Read the model definition and answer for the solid it produces. Units are mm, in the model's axes. A direction names the side the tool comes from. Coordinates: 2 decimals unless noted, no trailing zeros. Loops run counter-clockwise (first coordinate to the right, second up) from the corner with the lowest first, then second, coordinate; pieces in that order, holes last. Notation, with made-up numbers: (31.5, 47) -> (50.5, 47) arc R21 ccw to (50.5, 73) -> close; hole circle Ø10 at (33, 78). An arc over 180 degrees is marked (long way). Answer as CSV lines item,"result".
```python
from build123d import *

# Parameters (mm, degrees)
PAD_DEPTH    = 0.5
PAD001_DEPTH = 2.6
FILLET_R     = 0.4
FILLET001_R  = 0.2


with BuildPart() as part:
    # Sketch → Pad (new body)
    with BuildSketch(Plane.XY):
        with BuildLine():
            ThreePointArc((-3.175, 2.175), (-5.35, 0), (-3.175, -2.175))
            Line((-3.175, -2.175), (3.175, -2.175))
            ThreePointArc((3.175, -2.175), (5.35, 0), (3.175, 2.175))
            Line((-3.175, 2.175), (3.175, 2.175))
        make_face()
    extrude(amount=PAD_DEPTH)

    # Sketch001 (on Face6 of Pad) → Pad001 (join)
    with BuildSketch(Plane.XY.offset(0.5)):
        with BuildLine():
            ThreePointArc((-3.175, 1.69), (-4.865, 0), (-3.175, -1.69))
            Line((-3.175, -1.69), (3.175, -1.69))
            ThreePointArc((3.175, -1.69), (4.865, 0), (3.175, 1.69))
            Line((-3.175, 1.69), (3.175, 1.69))
        make_face()
    extrude(amount=PAD001_DEPTH)

    # Fillet
    fillet_edges = [part.edges().sort_by_distance(p)[0] for p in [
        (0, -1.69, 3.1),
    ]]
    fillet(fillet_edges, radius=FILLET_R)

    # Fillet001
    fillet001_edges = [part.edges().sort_by_distance(p)[0] for p in [
        (-5.35, 0, 0.5),
        (-5.35, 0, 0),
    ]]
    fillet(fillet001_edges, radius=FILLET001_R)


solid = part.part
```
Q1. Given pin 1 Ø1.5 at (x, z) = (-2, 2.5) entering from -Y; pin 2 Ø0.7 at (x, z) = (-1.5, 1.5) entering from +Y, each flat-ended and moving along its own axis, determine where each tip first touches the part or whether it passes through.
Results:
pin 1,"stops at y = -1.69"
pin 2,"stops at y = 1.69"
Q2. A cutting plane is placed at C-C, the plane z = 0.7. Write down the section's boundary in (x, y) (3 decimals), and give its area (3 significant figures).
Results:
outline,"(-3.175, -1.69) -> (3.175, -1.69) arc R1.69 ccw to (3.175, 1.69) -> (-3.175, 1.69) arc R1.69 ccw to start"
area,"30.4 mm²"
Q3. A cutting plane is placed at B-B, the plane y = 0. Write down the section's boundary in (x, z) (3 decimals), and give its area (3 significant figures).
Results:
outline,"(-5.35, 0.2) arc R0.2 ccw to (-5.15, 0) -> (5.15, 0) arc R0.2 ccw to (5.35, 0.2) -> (5.35, 0.3) arc R0.2 ccw to (5.15, 0.5) -> (4.865, 0.5) -> (4.865, 2.7) arc R0.4 ccw to (4.465, 3.1) -> (-4.465, 3.1) arc R0.4 ccw to (-4.865, 2.7) -> (-4.865, 0.5) -> (-5.15, 0.5) arc R0.2 ccw to (-5.35, 0.3) -> close"
area,"30.5 mm²"
Q4. A cutting plane is placed at A-A, the plane x = -0.75. Write down the section's boundary in (y, z) (3 decimals).
Results:
outline,"(-2.175, 0.2) arc R0.2 ccw to (-1.975, 0) -> (1.975, 0) arc R0.2 ccw to (2.175, 0.2) -> (2.175, 0.3) arc R0.2 ccw to (1.975, 0.5) -> (1.69, 0.5) -> (1.69, 2.7) arc R0.4 ccw to (1.29, 3.1) -> (-1.29, 3.1) arc R0.4 ccw to (-1.69, 2.7) -> (-1.69, 0.5) -> (-1.975, 0.5) arc R0.2 ccw to (-2.175, 0.3) -> close"
Q5. For faces 1 (the face through (0, 1.69, 2)), 2 (the face through (0, -1.69, 2)), 3 (the face through (4.865, -0.037, 1.585)), determine the directions among +Z, -Z, +X, -X, +Y, -Y from which every point of the face is accessible in a straight line to the end or side of a thin tool.
Results:
face 1,"+Z, +X, -X, +Y"
face 2,"+Z, +X, -X, -Y"
face 3,"+Z, +X"
Q6. Find the intervals of material crossed by probe 1 along Y at (x, z) = (0.5, 1.3); probe 2 along Z at (x, y) = (3.25, 1.9); probe 3 along Z at (x, y) = (-4.5, 0.2), in increasing order. Write a range as [from, to].
Results:
probe 1,"y = [-1.69, 1.69]"
probe 2,"z = [0, 0.5]"
probe 3,"z = [0, 3.1]"
Q7. A cutting plane is placed at D-D, the plane z = 2.8. Write down the section's boundary in (x, y) (3 decimals), and give its area (3 significant figures).
Results:
outline,"(-3.175, -1.677) -> (3.175, -1.677) arc R1.677 ccw to (3.175, 1.677) -> (-3.175, 1.677) arc R1.677 ccw to start"
area,"30.1 mm²"
